Check sheet for the modelled part. Datum: model origin and axes. Units: mm. A direction names the side the tool comes from. Give positions to 0.01 mm unless a question says otherwise; leave off trailing zeros. Loops run counter-clockwise (first coordinate to the right, second up) from the corner with the lowest first, then second, coordinate; pieces in that order, holes last. Notation, with made-up numbers: (55, -30) -> (84, -30) arc R20 cw to (84, -19) -> close; hole circle Ø9 at (23.25, 64.25). An arc over 180 degrees is marked (long way). Write each question's results on one line, items separated by ' | '. Start each with the question number.
Item 1: Cross-section at A-A on z = -17. Enter the section's corners in (x, y), then the cut area to 3 significant figures.
Item 2: Cross-section at C-C on x = 2.75. Enter the section's corners in (y, z).
Item 3: Access from +Z, -Z, +X, -X, +Y, -Y to the whole of each face (thin tool, end or side, straight path). Record for faces 5 (the face through (0, 3, -11)), 6 (the face through (-0.05, -3.77, 10.7)), 7 (the face through (-0.62, 16.97, -15.16)).
Item 4: Scan lines: line 1 along Y through (x, z) = (0, -18.75); line 2 along X through (y, z) = (-15, -18); line 3 along Y through (x, z) = (1.75, -13.5). Record each from-to range of solid material in increasing order.
Item 5: Cross-section at B-B on y = 0. Enter the section's corners in (x, z).
Item 6: Mould release check, pull along Z, two halves, no side actions. Record for faces 1 (the face through (-0.13, -4.83, 6.89)), 2 (the face through (0, -3, -11)), 3 (the face through (-0.1, -12.7, -22)), 4 (the face through (-0.098, -0.867, 3.905)): pulls with the +Z half, pulls with the -Z half, needs draft (parallel to the pull), parting line crosses it, or undercut.
Item 7: Cross-section at D-D on z = 3. Enter the section's corners in (x, y), then the cut area to 3 significant figures.
Item 8: Gauge pin test, flat ends, axial feed: pin 1 Ø4 at (x, z) = (-3, 2) entering from -Y; pin 2 Ø3.5 at (x, y) = (0, 15) entering from +Z; pin 3 Ø5 at (x, y) = (0, -15) entering from +Z. Record the tip position at first contact, or that the pin passes through.
Autodesk Inventor part; units mm, degrees
ref_plane "Work Plane1" through (16, 0, 0) normal (1, 0, 0) x (0, 0, -1)
ref_plane "Work Plane2" through (19.5, 0, 0) normal (1, 0, 0) x (0, 0, -1)
ref_plane "YZ Plane" through (0, 0, 0) normal (1, 0, 0) x (0, 1, 0)
sketch "Sketch1" plane through (0, 0, 0) normal (1, 0, 0) x (0, 1, 0)
  circle A0 centre (0, 0) radius 4
  line L0 (0, 0) -> (0, -22) construction
  line L1 (-10, -22) -> (-20, -22)
  line L2 (-20, -22) -> (-20, -19.8078)
  line L3 (10, -22) -> (20, -22)
  line L4 (20, -22) -> (20, -19.6315)
  line L5 (0, -9.2) -> (3, -9.2)
  line L6 (3, -9.2) -> (3, -12.4606)
  line L7 (0, -9.2) -> (-3, -9.2)
  line L8 (-3, -9.2) -> (-3, -12.4606)
  arc A1 (10, -22) -> (3, -12.4606) centre (0, -22) ccw
  arc A2 (-3, -12.4606) -> (-10, -22) centre (0, -22) ccw
  arc A3 (-19.9864, -19.6315) -> (-20, -19.8078) centre (-18.8527, -19.8078) ccw
  arc A4 (20, -19.6315) -> (19.8774, -18.0974) centre (10.3433, -19.6315) ccw
  line L9 (-19.9864, -19.6315) -> (-16, 6)
  line L10 (16, 6) -> (19.8774, -18.0974)
  line L11 (0, 14) -> (-10, 14)
  line L12 (-10, 14) -> (-16, 6)
  line L13 (0, 14) -> (10, 14)
  line L14 (10, 14) -> (16, 6)
  point P0 (-20, -12)
  point P1 (20, -12)
  dimension "d0" = 8
  dimension "d2" = 22
  dimension "d4" = 20
  dimension "d5" = 10
  dimension "d13" = 12.8
  dimension "d26" = 10
  dimension "d73" = 10
  dimension "d74" = 8
  dimension "d76" = 10
  dimension "d107" = 6
  dimension "d119" = 6
  dimension "d122" = 14
extrude "Extrusion1" add sketch "Sketch1" along normal mid plane 14
sketch "Sketch2" plane through (7, -10, -22) normal (0, 0, -1) x (-1, 0, 0)
  line L0 (14, 0) -> (14, -10)
  line L1 (7, 10) -> (-4.9056, 10) construction
  line L2 (14, 20) -> (0, 20)
  line L3 (0, 30) -> (0, 20)
  line L4 (0, 30) -> (14, 30)
  line L5 (14, 20) -> (14, 30)
  line L6 (0, -10) -> (0, 0)
  line L7 (14, 0) -> (0, 0)
  line L8 (0, -10) -> (14, -10)
  point P0 (5, 26.5)
  point P1 (5, -6.5)
  dimension "d46" = 5
  dimension "d48" = 3.5
  dimension "d50" = 5
  dimension "d51" = 3.5
ref_plane "Work Plane1" through (16, 0, 0) normal (1, 0, 0) x (0, 0, -1)
sketch "Sketch7" plane through (-7, 0, 0) normal (-1, 0, 0) x (0, 0, 1)
  circle A0 centre (0, 0) radius 4
  circle A1 centre (0, 0) radius 14.25
  dimension "d52" = 28.5
sketch "Sketch10" plane through (-7, -10, 14) normal (0, 0, 1) x (1, 0, 0)
  line L0 (0, 0) -> (14, 0)
  line L1 (14, 20) -> (14, 0)
  line L2 (0, 20) -> (14, 20)
  line L3 (0, 0) -> (0, 20)
  point P0 (7, 10)
sketch "Sketch15" plane through (7, -10, -22) normal (0, 0, -1) x (-1, 0, 0)
  line L0 (14, 0) -> (0, 0)
  line L1 (0, -10) -> (0, 0)
  line L2 (0, -10) -> (14, -10)
  line L3 (14, 0) -> (14, -10)
  point P0 (7, 10)
sketch "Sketch16" plane through (7, -10, -22) normal (0, 0, -1) x (-1, 0, 0)
  line L0 (0, -10) -> (14, -10)
  line L1 (14, 0) -> (14, -10)
  line L2 (7, -10) -> (7, 30.0311)
  line L3 (4.3309, -5) -> (12.7149, -5)
  line L4 (3.2036, 25) -> (11.1649, 25)
  line L5 (14, 30) -> (0, 30)
  line L6 (0, 20) -> (0, 30)
  line L7 (14, 20) -> (0, 20)
  line L8 (14, 30) -> (14, 20)
  point P0 (7, 10)
  point P1 (7, 25)
  point P2 (7, -5)
  dimension "d110" = 5
  dimension "d111" = 5
hole "Hole13" at (0, -15, -22) at (0, 15, -22) direction (0, 0, 1) diameter 4.134 depth 13.5 tip angle 118
ref_plane "Work Plane2" through (19.5, 0, 0) normal (1, 0, 0) x (0, 0, -1)
sketch "Sketch17" plane through (19.5, 0, 0) normal (1, 0, 0) x (0, 0, -1)
  point P0 (0, 0)
  point P1 (0, 0)
sketch "Sketch18" plane through (-7, -10, 14) normal (0, 0, 1) x (1, 0, 0)
  circle A0 centre (7, 15) radius 1.5
  line L0 (0, 0) -> (14, 0)
  line L1 (14, 20) -> (14, 0)
  line L2 (0, 20) -> (14, 20)
  line L3 (0, 0) -> (0, 20)
  circle A1 centre (7, 5) radius 1.5
  point P0 (7, 10)
  dimension "d132" = 7
hole "Hole14" at (0, 5, 14) at (0, -5, 14) direction (0, 0, -1) diameter 2.459 depth 6.5 tip angle 118
properties part number "2DOF-150-18-LEVS-01" material "Stainless Steel"
Answer sheet:
1) outline: (-7, -19.58) -> (7, -19.58) -> (7, -8.66) -> (-7, -8.66) -> close; (-7, 8.66) -> (7, 8.66) -> (7, 19.7) -> (-7, 19.7) -> close; hole circle Ø4.13 at (0, -15); hole circle Ø4.13 at (0, 15) | area: 281 mm²
2) outline: (-20, -22) -> (-10, -22) arc R10 cw to (-3, -12.46) -> (-3, -9.2) -> (3, -9.2) -> (3, -12.46) arc R10 cw to (10, -22) -> (20, -22) -> (20, -19.63) arc R9.66 ccw to (19.88, -18.1) -> (16, 6) -> (10, 14) -> (-10, 14) -> (-16, 6) -> (-19.99, -19.63) arc R1.14 ccw to (-20, -19.81) -> close; hole circle Ø8 at (0, 0)
3) face 5: -Z, +X, -X | face 6: +Z | face 7: -Z
4) line 1: y = -19.85 to -17.07, -12.93 to -9.46, 9.46 to 12.93, 17.07 to 19.96 | line 2: x = -7 to -2.07, 2.07 to 7 | line 3: y = -19.03 to -16.1, -13.9 to -5.27, 5.27 to 13.9, 16.1 to 19.14
5) outline: (-7, -9.2) -> (7, -9.2) -> (7, -4) -> (-7, -4) -> close; (-7, 4) -> (7, 4) -> (7, 14) -> (-7, 14) -> close
6) face 1: pulls with the +Z half | face 2: needs draft | face 3: pulls with the -Z half | face 4: undercut
7) outline: (-7, -16.47) -> (7, -16.47) -> (7, -2.65) -> (-7, -2.65) -> close; (-7, 2.65) -> (7, 2.65) -> (7, 16.48) -> (-7, 16.48) -> close | area: 387 mm²
8) pin 1: stops at y = -16.93 | pin 2: stops at z = 9.67 | pin 3: stops at z = 10.67
